```python
from build123d import *

# Parameters (mm, degrees)
SKIZZE1_W                       = 35
SKIZZE1_H                       = 35
SKIZZE1_W_2                     = 31
SKIZZE1_H_2                     = 31
AUFSATZ_LINEAR_AUSTRAGEN1_DEPTH = 185
SKIZZE6_W                       = 70
SKIZZE6_H                       = 31
SCHNITT_LINEAR_AUSTRAGEN1_DEPTH = 190.093230974
SKIZZE7_R                       = 3.15
SCHNITT_LINEAR_AUSTRAGEN2_DEPTH = 190.093230974
VERRUNDUNG1_R                   = 10
SKIZZE10_W                      = 39.330921978
SKIZZE10_H                      = 37.025640666
SCHNITT_LINEAR_AUSTRAGEN3_DEPTH = 25
SKIZZE11_R                      = 5
SCHNITT_LINEAR_AUSTRAGEN4_DEPTH = 190.093230974


with BuildPart() as part:
    # Skizze1 → Aufsatz-Linear austragen1 (new body)
    with BuildSketch(Plane.XY):
        Rectangle(SKIZZE1_W, SKIZZE1_H)
        Rectangle(SKIZZE1_W_2, SKIZZE1_H_2, mode=Mode.SUBTRACT)
    extrude(amount=AUFSATZ_LINEAR_AUSTRAGEN1_DEPTH)

    # Skizze6 → Schnitt-Linear austragen1 (cut, through all)
    with BuildSketch(Plane(origin=(17.5, 0, 0), x_dir=(0, 0, -1), z_dir=(1, 0, 0))):
        with Locations((-150, 0)):
            Rectangle(SKIZZE6_W, SKIZZE6_H)
    extrude(amount=-SCHNITT_LINEAR_AUSTRAGEN1_DEPTH, mode=Mode.SUBTRACT)

    # Skizze7 → Schnitt-Linear austragen2 (cut, through all)
    with BuildSketch(Plane.XZ.offset(17.5)):
        with Locations(Location((0, 170, 0), (0, 0, 270))):
            Circle(SKIZZE7_R)
    extrude(amount=-SCHNITT_LINEAR_AUSTRAGEN2_DEPTH, mode=Mode.SUBTRACT)

    # Verrundung1
    verrundung1_edges = [part.edges().sort_by_distance(p)[0] for p in [
        (-17.5, 16.5, 185),
        (-17.5, -16.5, 185),
        (17.5, 16.5, 185),
        (17.5, -16.5, 185),
    ]]
    fillet(verrundung1_edges, radius=VERRUNDUNG1_R)

    # Skizze10 → Schnitt-Linear austragen3 (cut)
    with BuildSketch(Plane(origin=(0, 0, 0), x_dir=(-1, 0, 0), z_dir=(0, 0, -1))):
        Rectangle(SKIZZE10_W, SKIZZE10_H)
    extrude(amount=-SCHNITT_LINEAR_AUSTRAGEN3_DEPTH, mode=Mode.SUBTRACT)

    # Skizze11 → Schnitt-Linear austragen4 (cut, through all)
    with BuildSketch(Plane(origin=(0, 17.5, 0), x_dir=(1, 0, 0), z_dir=(0, 1, 0))):
        with Locations(Location((10.5, -40, 0), (0, 0, 270))):
            Circle(SKIZZE11_R)
        with Locations(Location((-10.5, -67, 0), (0, 0, 270))):
            Circle(SKIZZE11_R)
    extrude(amount=-SCHNITT_LINEAR_AUSTRAGEN4_DEPTH, mode=Mode.SUBTRACT)


solid = part.part
```
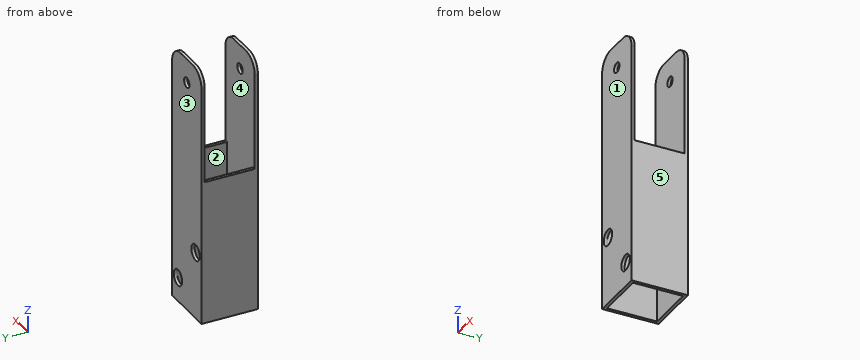
The listing builds one solid part. Answer for the finished solid, in the listing's coordinates (mm). Face numbers are marked on the shaded views. A direction names the side the tool comes from. Give positions to 0.01 mm unless a question says otherwise; leave off trailing zeros. Loops run counter-clockwise (first coordinate to the right, second up) from the corner with the lowest first, then second, coordinate; pieces in that order, holes last. Notation, with made-up numbers: (68.5, 81.5) - (82.5, 81.5) arc R20 ccw to (82.5, 116.5) - close; hole circle Ø11 at (27, -1). An arc over 180 degrees is marked (long way). Answer as CSV lines item,"result". Start each with the question number.
Item 1: For the marked faces 1 and 2, determine the directions among +Z, -Z, +X, -X, +Y, -Y from which every point of the face is accessible in a straight line to the end or side of a thin tool.
Item 2: A cutting plane is placed at A-A on y = 8.5. Determine the outline of the cut face in (x, z), then the cut area to 3 significant figures.
Item 3: A cutting plane is placed at B-B on z = 170. Determine the outline of the cut face in (x, y), then the cut area to 3 significant figures.
Item 4: The mould has two halves that part along X. Classify the marked faces 3, 4 and 5: +X half, -X half, draft (parallel to the pull), parting line (faces both ways), or undercut.
Item 5: Find the intervals of material crossed by line 1 (X direction, y = -3, z = 93.5); line 2 (X direction, y = 16, z = 40), in increasing order. Write a range as from..to.
Item 6: A cutting plane is placed at C-C on x = 0. Determine the outline of the cut face in (y, z), then the cut area to 3 significant figures.
Item 7: A cutting plane is placed at D-D on z = 112.5. Determine the outline of the cut face in (x, y), then the cut area to 3 significant figures.
Item 8: This flat-tipped pin is pushed along its axis until it touches: pin 1 (2 mm diameter, centred on x = -17, y = 0, fed in from +Z). Where does it stop, or does it pass through?
Found:
1,face 1,"+Z, -Z, +X, -X, -Y"
1,face 2,"+Z, -Z"
2,outline,"(-17.5, 25) - (-15.5, 25) - (-15.5, 115) - (-17.5, 115) - close; (15.5, 25) - (17.5, 25) - (17.5, 115) - (15.5, 115) - close"
2,area,"360 mm^2"
3,outline,"(-17.5, -17.5) - (-3.15, -17.5) - (-3.15, -15.5) - (-17.5, -15.5) - close; (-17.5, 15.5) - (-3.15, 15.5) - (-3.15, 17.5) - (-17.5, 17.5) - close; (3.15, -17.5) - (17.5, -17.5) - (17.5, -15.5) - (3.15, -15.5) - close; (3.15, 15.5) - (17.5, 15.5) - (17.5, 17.5) - (3.15, 17.5) - close"
3,area,"115 mm^2"
4,face 3,"draft"
4,face 4,"undercut"
4,face 5,"+X half"
5,line 1,"x = -17.5..-15.5, 15.5..17.5"
5,line 2,"x = -17.5..5.5, 15.5..17.5"
6,outline,"(-17.5, 25) - (-15.5, 25) - (-15.5, 166.85) - (-17.5, 166.85) - close; (-17.5, 173.15) - (-15.5, 173.15) - (-15.5, 185) - (-17.5, 185) - close; (15.5, 25) - (17.5, 25) - (17.5, 166.85) - (15.5, 166.85) - close; (15.5, 173.15) - (17.5, 173.15) - (17.5, 185) - (15.5, 185) - close"
6,area,"615 mm^2"
7,outline,"(-17.5, -17.5) - (17.5, -17.5) - (17.5, 17.5) - (-17.5, 17.5) - close; hole (-15.5, -15.5) - (15.5, -15.5) - (15.5, 15.5) - (-15.5, 15.5) - close"
7,area,"264 mm^2"
8,pin 1,"stops at z = 115"
